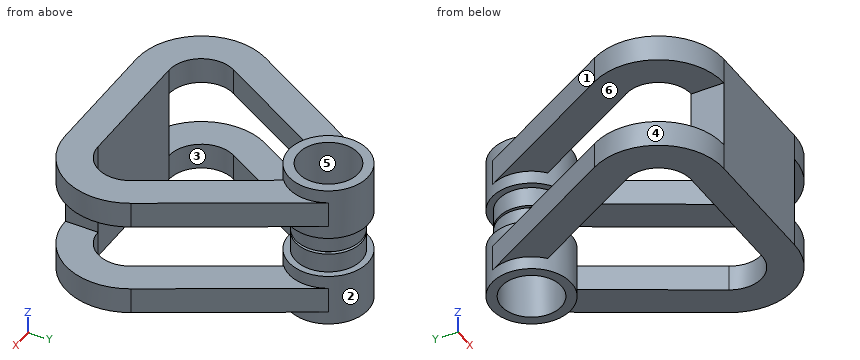
from build123d import *

# Parameters (mm, degrees)
SKETCH1_R                = 5.1
SKETCH1_R_2              = 4.6
EXTRUDE_THIN1_DEPTH      = 11
SKETCH2_R                = 6.1
SKETCH2_R_2              = 5.1
BOSS_EXTRUDE2_DEPTH      = 8
BOSS_EXTRUDE3_DEPTH      = 2
BOSS_EXTRUDE3_DEPTH_BACK = 2
SKETCH4_W                = 19.308386588
SKETCH4_H                = 5
BOSS_EXTRUDE4_DEPTH      = 5.2


with BuildPart() as part:
    # Sketch1 → Extrude-Thin1 (new body)
    with BuildSketch(Plane.XY):
        Circle(SKETCH1_R)
        Circle(SKETCH1_R_2, mode=Mode.SUBTRACT)
    extrude(amount=EXTRUDE_THIN1_DEPTH)

    # Sketch2 → Boss-Extrude2 (add)
    with BuildSketch(Plane.XY.offset(11)):
        Circle(SKETCH2_R)
        Circle(SKETCH2_R_2, mode=Mode.SUBTRACT)
    extrude(amount=-BOSS_EXTRUDE2_DEPTH)

    # Sketch3 → Boss-Extrude3 (add, two sides)
    with BuildSketch(Plane.XY.offset(7)) as boss_extrude3_sk:
        with BuildLine():
            Line((5.305614658, 3.010058653), (18.351922243, -19.9857327))
            ThreePointArc((18.351922243, -19.9857327), (18.2955249, -29.952887404), (9.654193294, -34.920255082))
            Line((9.654193294, -34.920255082), (-9.654193294, -34.920255082))
            ThreePointArc((-9.654193294, -34.920255082), (-18.2955249, -29.952887404), (-18.351922243, -19.9857327))
            Line((-18.351922243, -19.9857327), (-5.305614658, 3.010058653))
            ThreePointArc((-5.305614658, 3.010058653), (-6.002878674, -1.084180624), (-3.917463614, -4.675839907))
            Line((-3.917463614, -4.675839907), (-14.003057769, -22.452993891))
            ThreePointArc((-14.003057769, -22.452993891), (-13.974859097, -27.436571243), (-9.654193294, -29.920255082))
            Line((-9.654193294, -29.920255082), (9.654193294, -29.920255082))
            ThreePointArc((9.654193294, -29.920255082), (13.974859097, -27.436571243), (14.003057769, -22.452993891))
            Line((14.003057769, -22.452993891), (3.917463614, -4.675839907))
            ThreePointArc((3.917463614, -4.675839907), (6.002878674, -1.084180624), (5.305614658, 3.010058653))
        make_face()
    extrude(amount=BOSS_EXTRUDE3_DEPTH)
    extrude(boss_extrude3_sk.sketch, amount=-BOSS_EXTRUDE3_DEPTH_BACK)

    # Sketch4 → Boss-Extrude4 (add)
    with BuildSketch(Plane(origin=(0, 0, -0.2), x_dir=(-1, 0, 0), z_dir=(0, 0, -1))):
        with Locations((0, -32.420255082)):
            Rectangle(SKETCH4_W, SKETCH4_H)
    extrude(amount=-BOSS_EXTRUDE4_DEPTH)

    # Mirror3: part across plane


with BuildPart() as part_1:
    add(part.part)
    add(part.part.mirror(Plane(origin=(0, 0, -0.2), x_dir=(1, 0, 0), z_dir=(0, 0, -1))))


solid = part_1.part
CAD build for the part. Positions are in the model's coordinates, mm. Face numbers are marked on the shaded views. A direction names the side the tool comes from. Give positions to 0.01 mm unless a question says otherwise; leave off trailing zeros. Loops run counter-clockwise (first coordinate to the right, second up) from the corner with the lowest first, then second, coordinate; pieces in that order, holes last. Notation, with made-up numbers: M 8.25,-24.5 L 38.25,-24.5 A19 ccw 38.25,12.5 Z; hole C 75,89.25 d3. An arc over 180 degrees is marked long. Write each question's results on one line, items separated by ' | '.
Q1. Which spindle directions (+Z, -Z, +X, -X, +Y, -Y) get a long thin tool onto all of the face, cutting with end or side? Do the marked faces 1, 2 and 3. Say none if no direction does.
Geometry check:
face 1: +Z, -Z, -X, +Y | face 2: none | face 3: +Z, -Z
Q2. Band-saw the part on B-B on x = 0. Write the cut outline in (y, z), and give its area (3 significant figures).
Geometry check:
outline: M -34.92,-9.4 L -29.92,-9.4 L -29.92,9 L -34.92,9 Z; M -6.1,-11.4 L -4.6,-11.4 L -4.6,-0.4 L -5.1,-0.4 L -5.1,-3.4 L -6.1,-3.4 Z; M -6.1,3 L -5.1,3 L -5.1,0 L -4.6,0 L -4.6,11 L -6.1,11 Z; M 4.6,-11.4 L 6.1,-11.4 L 6.1,-3.4 L 5.1,-3.4 L 5.1,-0.4 L 4.6,-0.4 Z; M 4.6,0 L 5.1,0 L 5.1,3 L 6.1,3 L 6.1,11 L 4.6,11 Z | area: 146 mm²
Q3. Probe probe 1 along Z at (x, y) = (-7, -7); probe 2 along Y at (x, z) = (0, 5.25); probe 3 along Y at (x, z) = (4, -4.25). List the from-to ranges inside material, lowest first.
Geometry check:
probe 1: z = -9.4 to -5.4, 5 to 9 | probe 2: y = -34.92 to -29.92, -6.1 to -4.6, 4.6 to 6.1 | probe 3: y = -34.92 to -29.92, -4.61 to -2.27, 2.27 to 4.61
Q4. Mould opens along X. For the marked faces 4, 5 and 6 say: pulls with the +X half, pulls with the -X half, needs draft (parallel to the pull), parting line crosses it, or undercut.
Geometry check:
face 4: pulls with the -X half | face 5: undercut | face 6: needs draft
Q5. Flat gauge pins, fed straight in: P1, Ø10, axis at y = -3, z = -6, coming from the +X side; P2, Ø2.5, axis at y = -32.5, z = 0, coming from the +X side; P3, Ø8, axis at y = -29.5, z = -8.5, coming from the -X side; P4, Ø4.5, axis at x = -15, y = -6.5, coming from the -Z side. Where does each tip first touch, or does it go through?
Geometry check:
P1: stops at x = 11.55 | P2: stops at x = 9.65 | P3: stops at x = -19.64 | P4: passes through
Q6. Band-saw the part on A-A on z = 1.25. Write the cut outline in (x, y), and give its area (3 significant figures).
Geometry check:
outline: M -9.65,-34.92 L 9.65,-34.92 L 9.65,-29.92 L -9.65,-29.92 Z; C 0,0 d10.2; hole C 0,0 d9.2 | area: 112 mm²
Q7. Band-saw the part on C-C on x = -12. Write the cut outline in (y, z).
Geometry check:
outline: M -34.64,-9.4 L -29.34,-9.4 L -29.34,-5.4 L -34.64,-5.4 Z; M -34.64,5 L -29.34,5 L -29.34,9 L -34.64,9 Z; M -18.92,-9.4 L -8.79,-9.4 L -8.79,-5.4 L -18.92,-5.4 Z; M -18.92,5 L -8.79,5 L -8.79,9 L -18.92,9 Z
Q8. Band-saw the part on D-D on x = 16. Write the cut outline in (y, z), and give its area (3 significant figures).
Geometry check:
outline: M -32.65,-9.4 L -15.84,-9.4 L -15.84,-5.4 L -32.65,-5.4 Z; M -32.65,5 L -15.84,5 L -15.84,9 L -32.65,9 Z | area: 134 mm²
